Part model, mm, in its own coordinate system. A direction names the side the tool comes from. Round coordinates to 2 decimals unless told otherwise and drop trailing zeros. Order: outer loops, then holes, each group sorted by start corner. A loop starts at its lowest first (then second) coordinate and runs counter-clockwise, first axis right, second up. Notation, with made-up numbers: M 75,46.25 L 93,46.25 A19 cw 93,51.25 Z; hole C 37.5,26 d1. An arc over 180 degrees is marked long. One line per question, with ' | ' between items.
from build123d import *

# Parameters (mm, degrees)
SKETCH1_W                = 90
SKETCH1_H                = 190
BOSS_EXTRUDE1_DEPTH      = 5
SKETCH2_W                = 10
SKETCH2_H                = 30
BOSS_EXTRUDE2_DEPTH      = 5
CHAMFER1_SIZE            = 2
SKETCH3_W                = 16
SKETCH3_H                = 34
CUT_EXTRUDE1_DEPTH       = 50
SKETCH4_W                = 90
SKETCH4_H                = 42
CUT_EXTRUDE2_DEPTH       = 1
SKETCH7_W                = 15.1
SKETCH7_H                = 89.916335477
CUT_EXTRUDE7_DEPTH       = 1
CUT_EXTRUDE8_DEPTH       = 1
CUT_EXTRUDE9_DEPTH       = 110.886304879
CUT_EXTRUDE9_DEPTH_BACK  = 110.886304879
CUT_EXTRUDE10_DEPTH      = 110.886304879
CUT_EXTRUDE10_DEPTH_BACK = 110.886304879
BOSS_EXTRUDE4_START      = 5
SKETCH17_W               = 2.5
SKETCH17_H               = 8
BOSS_EXTRUDE4_DEPTH      = 13
BOSS_EXTRUDE5_DEPTH      = 3.1


with BuildPart() as part:
    # Sketch1 → Boss-Extrude1 (new body)
    with BuildSketch(Plane(origin=(0, 0, 0), x_dir=(1, 0, 0), z_dir=(0, 1, 0))):
        Rectangle(SKETCH1_W, SKETCH1_H)
    extrude(amount=BOSS_EXTRUDE1_DEPTH)

    # Sketch2 → Boss-Extrude2 (add)
    with BuildSketch(Plane(origin=(0, 0, 0), x_dir=(1, 0, 0), z_dir=(0, 1, 0))):
        with Locations((-50, -80)):
            Rectangle(SKETCH2_W, SKETCH2_H)
        with Locations((50, -80)):
            Rectangle(SKETCH2_W, SKETCH2_H)
    extrude(amount=BOSS_EXTRUDE2_DEPTH)

    # Chamfer1
    chamfer1_edges = [part.edges().sort_by_distance(p)[0] for p in [
        (-55, 2.5, 65),
        (-55, 2.5, 95),
        (55, 2.5, 95),
        (55, 2.5, 65),
    ]]
    chamfer(chamfer1_edges, length=CHAMFER1_SIZE)

    # Sketch3 → Cut-Extrude1 (cut)
    with BuildSketch(Plane(origin=(0, 5, 0), x_dir=(1, 0, 0), z_dir=(0, 1, 0))):
        with Locations((-25, -78)):
            Rectangle(SKETCH3_W, SKETCH3_H)
    extrude(amount=-CUT_EXTRUDE1_DEPTH, mode=Mode.SUBTRACT)

    # Sketch4 → Cut-Extrude2 (cut)
    with BuildSketch(Plane(origin=(0, 5, 0), x_dir=(1, 0, 0), z_dir=(0, 1, 0))):
        with Locations((0, 59.159820088)):
            Rectangle(SKETCH4_W, SKETCH4_H)
    extrude(amount=-CUT_EXTRUDE2_DEPTH, mode=Mode.SUBTRACT)

    # Sketch7 → Cut-Extrude7 (cut)
    with BuildSketch(Plane(origin=(0, 5, 0), x_dir=(1, 0, 0), z_dir=(0, 1, 0))):
        with Locations((37.45, -15.495273531)):
            Rectangle(SKETCH7_W, SKETCH7_H)
        with Locations((0.16773297, -15.495273531)):
            Rectangle(SKETCH7_W, SKETCH7_H)
    extrude(amount=-CUT_EXTRUDE7_DEPTH, mode=Mode.SUBTRACT)

    # Sketch8 → Cut-Extrude8 (cut)
    with BuildSketch(Plane(origin=(0, 5, 0), x_dir=(1, 0, 0), z_dir=(0, 1, 0))):
        Polygon((-34.9, -70.1), (-45.958578644, -70.1), (-47.9, -72.041421356), (-47.9, -87.958578644), (-45.958578644, -89.9), (-34.9, -89.9), (-34.9, -95.1), (-53.041421356, -95.1), (-55.1, -93.041421356), (-55.1, -66.958578644), (-53.041421356, -64.9), (-34.9, -64.9), align=None)
    cut_extrude8 = extrude(amount=-CUT_EXTRUDE8_DEPTH, mode=Mode.SUBTRACT)

    # Mirror1: Cut-Extrude8 across plane
    add(cut_extrude8.mirror(Plane(origin=(0, 0, 0), x_dir=(0, 0, 1), z_dir=(1, 0, 0))), mode=Mode.SUBTRACT)

    # Sketch14 → Cut-Extrude9 (cut, two sides: drawn at the far end of the back side and taken through both)
    with BuildSketch(Plane(origin=(0, 0, 0), x_dir=(1, 0, 0), z_dir=(0, 1, 0)).offset(-CUT_EXTRUDE9_DEPTH_BACK)):
        with BuildLine():
            Line((-45, 47.267125731), (-34.685032462, 30.799006468))
            ThreePointArc((-34.685032462, 30.799006468), (-34.351546651, 18.443044928), (-45, 12.166784925))
            Line((-45, 12.166784925), (-45, 47.267125731))
        make_face()
        with BuildLine():
            Line((45, 47.267125731), (45, 12.166784925))
            ThreePointArc((45, 12.166784925), (34.351546651, 18.443044928), (34.685032462, 30.799006468))
            Line((34.685032462, 30.799006468), (45, 47.267125731))
        make_face()
    extrude(amount=CUT_EXTRUDE9_DEPTH + CUT_EXTRUDE9_DEPTH_BACK, mode=Mode.SUBTRACT)

    # Sketch16 → Cut-Extrude10 (cut, two sides: drawn at the far end of the back side and taken through both)
    with BuildSketch(Plane(origin=(0, 0, 0), x_dir=(1, 0, 0), z_dir=(0, 1, 0)).offset(-CUT_EXTRUDE10_DEPTH_BACK)):
        with BuildLine():
            Line((-32.828659242, 95), (-32.828659242, 24.338125683))
            ThreePointArc((-32.828659242, 24.338125683), (-33.30195485, 27.699267678), (-34.685032462, 30.799006468))
            Line((-34.685032462, 30.799006468), (-45, 47.267125731))
            Line((-45, 47.267125731), (-45, 95))
            Line((-45, 95), (-32.828659242, 95))
        make_face()
        with BuildLine():
            Line((45, 95), (32.828659242, 95))
            Line((32.828659242, 95), (32.828659242, 24.338125683))
            ThreePointArc((32.828659242, 24.338125683), (33.30195485, 27.699267678), (34.685032462, 30.799006468))
            Line((34.685032462, 30.799006468), (45, 47.267125731))
            Line((45, 47.267125731), (45, 95))
        make_face()
    extrude(amount=CUT_EXTRUDE10_DEPTH + CUT_EXTRUDE10_DEPTH_BACK, mode=Mode.SUBTRACT)

    # Sketch17 → Boss-Extrude4 (add)
    with BuildSketch(Plane(origin=(0, 0, 0), x_dir=(1, 0, 0), z_dir=(0, 1, 0)).offset(BOSS_EXTRUDE4_START)):
        with Locations((-21.190023983, 84.159820088)):
            Rectangle(SKETCH17_W, SKETCH17_H)
        Polygon((-22.440023983, 94.999820088), (-22.440023983, 92.499820088), (18.940023983, 92.499820088), (19.940023983, 91.499820088), (19.940023983, 80.159820088), (22.440023983, 80.159820088), (22.440023983, 92.535353994), (19.975557889, 94.999820088), align=None)
    extrude(amount=BOSS_EXTRUDE4_DEPTH)

    # Sketch18 → Boss-Extrude5 (add)
    with BuildSketch(Plane(origin=(0, 5, 0), x_dir=(1, 0, 0), z_dir=(0, 1, 0))):
        Polygon((-12.599634528, 80.159820088), (-10.599634528, 80.159820088), (-6.108241837, 92.499820088), (-8.108241837, 92.499820088), align=None)
        Polygon((-3.108241837, 92.499820088), (-7.599634528, 80.159820088), (-5.599634528, 80.159820088), (-1.108241837, 92.499820088), align=None)
        Polygon((1.891758163, 92.499820088), (-2.599634528, 80.159820088), (-0.599634528, 80.159820088), (3.891758163, 92.499820088), align=None)
        Polygon((6.891758163, 92.499820088), (2.400365472, 80.159820088), (4.400365472, 80.159820088), (8.891758163, 92.499820088), align=None)
        Polygon((11.891758163, 92.499820088), (7.400365472, 80.159820088), (9.400365472, 80.159820088), (13.891758163, 92.499820088), align=None)
    extrude(amount=BOSS_EXTRUDE5_DEPTH)


solid = part.part
1) Probe line 1 (Z direction, x = -23, y = 4.25); line 2 (Z direction, x = 15.5, y = 16); line 3 (Y direction, x = 23, z = 63). List the from-to ranges inside material, lowest first. Write a range as [from, to].
The answers:
line 1: z = [-95, -80.16], [-38.16, 61] | line 2: z = [-95, -92.5] | line 3: y = [0, 5]
2) Saw through at C-C (x = -26). List the corners of the cut face in (y, z), plus the area to 3 significant figures.
The answers:
outline: M 0,-95 L 5,-95 L 5,-80.16 L 4,-80.16 L 4,-38.16 L 5,-38.16 L 5,61 L 0,61 Z | area: 738 mm²
3) Two-plate mould, pull along Z, no slides. Class faces 1 (the face through (-2, 11, -92.5)), 2 (the face through (-43, 2, 95)), 3 (the face through (0, 4, 15)), 4 (the face through (0, 2, -95)): released by +Z, released by -Z, zero draft, split by the parting line, or undercut.
The answers:
face 1: undercut | face 2: released by +Z | face 3: undercut | face 4: released by -Z
4) Which spindle directions (+Z, -Z, +X, -X, +Y, -Y) get a long thin tool onto all of the face, cutting with end or side? Do faces 5 (the face through (5, 8.1, -86)), 6 (the face through (37, 4, 25)), 7 (the face through (-8.4, 6.5, -86.2)). Say none if no direction does.
The answers:
face 5: +Z, +Y | face 6: +X, +Y | face 7: +Y
5) Drop flat-ended pins along their axis: pin 1 (0.8 mm diameter, centred on y = 4.5, z = 19, fed in from -X); pin 2 (2 mm diameter, centred on x = 39.5, z = 16.5, fed in from +Y); pin 3 (3.5 mm diameter, centred on x = -5, z = -84.5, fed in from +Y). Give the stop position or say it passes through.
The answers:
pin 1: stops at x = -45 | pin 2: stops at y = 4 | pin 3: stops at y = 8.1
6) Saw through at B-B (z = 14). List the corners of the cut face in (x, y).
The answers:
outline: M -45,0 L 45,0 L 45,4 L 29.9,4 L 29.9,5 L 7.72,5 L 7.72,4 L -7.38,4 L -7.38,5 L -45,5 Z
7) Saw through at A-A (y = 11.75). List the corners of the cut face in (x, z), plus the area to 3 significant figures.
The answers:
outline: M -22.44,-95 L 19.98,-95 L 22.44,-92.54 L 22.44,-80.16 L 19.94,-80.16 L 19.94,-91.5 L 18.94,-92.5 L -22.44,-92.5 Z; M -22.44,-88.16 L -19.94,-88.16 L -19.94,-80.16 L -22.44,-80.16 Z | area: 161 mm²
8) Saw through at D-D (x = -40). List the corners of the cut face in (y, z), plus the area to 3 significant figures.
The answers:
outline: M 0,-13.24 L 5,-13.24 L 5,64.9 L 4,64.9 L 4,70.1 L 5,70.1 L 5,89.9 L 4,89.9 L 4,95 L 0,95 Z | area: 531 mm²
